```python
from build123d import *

# Parameters (mm, degrees)
BOSS_EXTRUDE1_DEPTH = 25.4
SKETCH2_R           = 3.175
CUT_EXTRUDE1_DEPTH  = 25.4
SKETCH3_R           = 3.175
CUT_EXTRUDE2_DEPTH  = 25.4


with BuildPart() as part:
    # Sketch1 → Boss-Extrude1 (new body)
    with BuildSketch(Plane(origin=(0, 0, 0), x_dir=(1, 0, 0), z_dir=(0, 1, 0))):
        with BuildLine():
            Line((0, 0), (34.925, 0))
            ThreePointArc((34.925, 0), (37.17006403, -0.92993597), (38.1, -3.175))
            Line((38.1, -3.175), (38.1, -38.1))
            Line((38.1, -38.1), (36.195, -38.1))
            ThreePointArc((36.195, -38.1), (35.296974388, -37.728025612), (34.925, -36.83))
            Line((34.925, -36.83), (34.925, -9.525))
            ThreePointArc((34.925, -9.525), (33.065128061, -5.034871939), (28.575, -3.175))
            Line((28.575, -3.175), (1.27, -3.175))
            ThreePointArc((1.27, -3.175), (0.371974388, -2.803025612), (0, -1.905))
            Line((0, -1.905), (0, 0))
        make_face()
    extrude(amount=-BOSS_EXTRUDE1_DEPTH)

    # Sketch2 → Cut-Extrude1 (cut)
    with BuildSketch(Plane.ZY.offset(-34.925)):
        with Locations((30.48, -12.7)):
            Circle(SKETCH2_R)
        with Locations((13.97, -12.7)):
            Circle(SKETCH2_R)
    extrude(amount=-CUT_EXTRUDE1_DEPTH, mode=Mode.SUBTRACT)

    # Sketch3 → Cut-Extrude2 (cut)
    with BuildSketch(Plane.XY.offset(3.175)):
        with Locations((6.35, -12.7)):
            Circle(SKETCH3_R)
        with Locations((22.86, -12.7)):
            Circle(SKETCH3_R)
    extrude(amount=-CUT_EXTRUDE2_DEPTH, mode=Mode.SUBTRACT)


solid = part.part
```
Work out the finished part from the listing and answer in its coordinate system (mm). A direction names the side the tool comes from. Give positions to 0.01 mm unless a question says otherwise; leave off trailing zeros. Order: outer loops, then holes, each group sorted by start corner. A loop starts at its lowest first (then second) coordinate and runs counter-clockwise, first axis right, second up. Notation, with made-up numbers: (20.5, 13) -> (32.5, 13) arc R25 ccw to (32.5, 31) -> close; hole circle Ø3 at (18.5, 64). An arc over 180 degrees is marked (long way). Answer as CSV lines item,"result". Start each with the question number.
(1) Section B-B, the plane y = -12.7 is taken. Write down the section's boundary in (x, z) (3 decimals).
(2) Section D-D, the plane z = 12 is taken. Write down the section's boundary in (x, y) (3 decimals).
(3) Section A-A, the plane x = 22.86 is taken. Write down the section's boundary in (y, z) (3 decimals), plus the area to 3 significant figures.
(4) Section C-C, the plane y = -18.5 is taken. Write down the section's boundary in (x, z) (3 decimals), plus the area to 3 significant figures.
(5) For a pull along Y with two mould halves and no side action, classify faces 3 (the cylindrical face through (0.38, -12.52, 2.81)), 4 (the flat face through (35, -25.4, 8)), 5 (the cylindrical face through (3.83, -14.63, 1.61)) as released by +Y, released by -Y, zero draft, split by the parting line, or undercut.
(6) Consider line 1 along Z through (x, y) = (36, -13.25); line 2 along Y through (x, z) = (36, 30.48) (3 decimals); line 3 along Z through (x, y) = (22, -19.5) (3 decimals). Determine where each line is inside the solid, lowest interval first.
(7) Each of these flat-tipped pins is pushed along its axis until it touches: pin 1 Ø12.5 at (y, z) = (-9, 23.5) entering from -X (3 decimals); pin 2 Ø12.5 at (x, y) = (12.5, -10) entering from +Z (3 decimals); pin 3 Ø8 at (x, z) = (29, 18) entering from +Y. Where does it stop, or does it pass through?
(8) Which of the six approach directions +Z, -Z, +X, -X, +Y, -Y give full straight-line access (tool end or side, diameter ignored) to faces 1 (the flat face through (15, -13, 3.175)), 2 (the cylindrical face through (36.49, -14.63, 11.45))?
Entries:
1,outline,"(0, 0) -> (3.175, 0) -> (3.175, 3.175) -> (1.27, 3.175) arc R1.27 ccw to (0, 1.905) -> close; (9.525, 0) -> (19.685, 0) -> (19.685, 3.175) -> (9.525, 3.175) -> close; (26.035, 0) -> (34.925, 0) arc R3.175 ccw to (38.1, 3.175) -> (38.1, 10.795) -> (34.925, 10.795) -> (34.925, 9.525) arc R6.35 cw to (28.575, 3.175) -> (26.035, 3.175) -> close; (34.925, 17.145) -> (38.1, 17.145) -> (38.1, 27.305) -> (34.925, 27.305) -> close; (34.925, 33.655) -> (38.1, 33.655) -> (38.1, 38.1) -> (36.195, 38.1) arc R1.27 ccw to (34.925, 36.83) -> close"
2,outline,"(34.925, -25.4) -> (38.1, -25.4) -> (38.1, -15.19) -> (34.925, -15.19) -> close; (34.925, -10.21) -> (38.1, -10.21) -> (38.1, 0) -> (34.925, 0) -> close"
3,outline,"(-25.4, 0) -> (-15.875, 0) -> (-15.875, 3.175) -> (-25.4, 3.175) -> close; (-9.525, 0) -> (0, 0) -> (0, 3.175) -> (-9.525, 3.175) -> close"
3,area,"60.5 mm²"
4,outline,"(0, 0) -> (34.925, 0) arc R3.175 ccw to (38.1, 3.175) -> (38.1, 38.1) -> (36.195, 38.1) arc R1.27 ccw to (34.925, 36.83) -> (34.925, 9.525) arc R6.35 cw to (28.575, 3.175) -> (1.27, 3.175) arc R1.27 ccw to (0, 1.905) -> close"
4,area,"238 mm²"
5,face 3,"zero draft"
5,face 4,"released by -Y"
5,face 5,"undercut"
6,line 1,"0.19 to 10.84, 17.1 to 27.35, 33.61 to 38.08"
6,line 2,"-25.4 to -15.875, -9.525 to 0"
6,line 3,"0 to 3.175"
7,pin 1,"x = 34.925"
7,pin 2,"z = 3.175"
7,pin 3,"through"
8,face 1,"+Z, -X, +Y, -Y"
8,face 2,"+X, -X"
